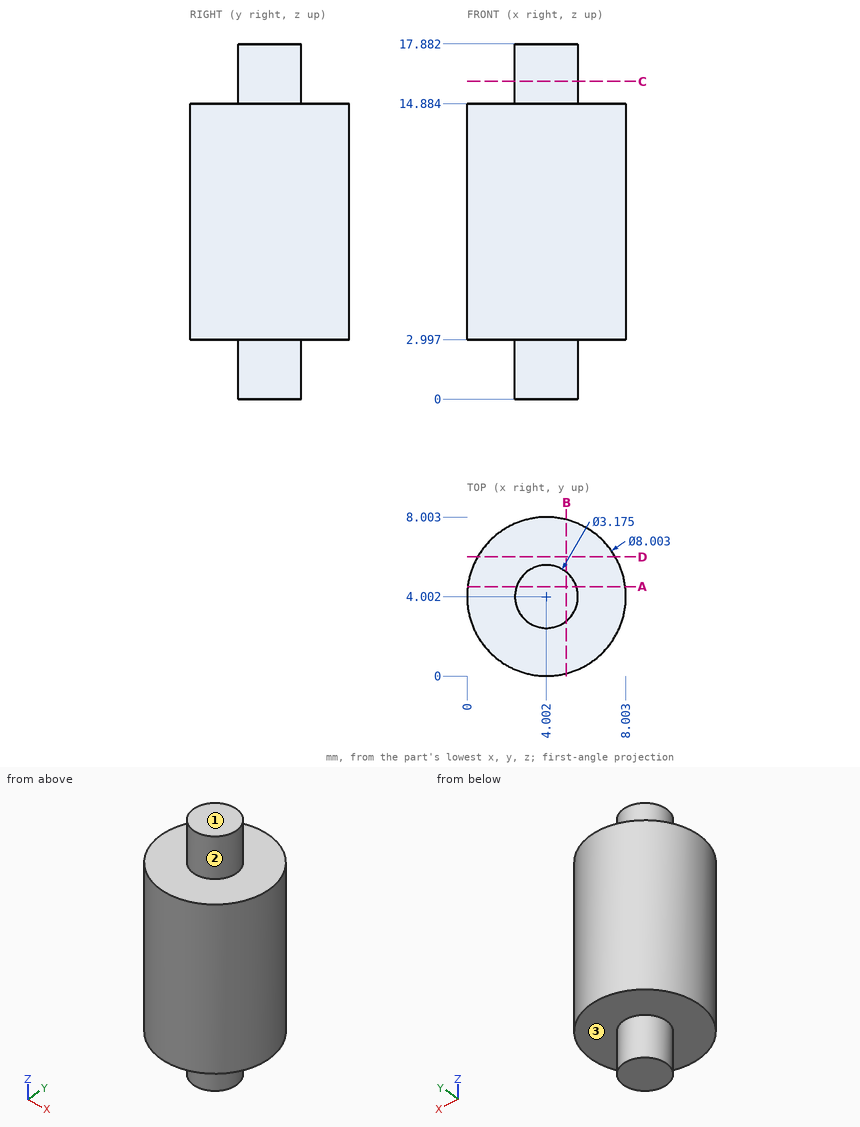
Verification items for this drawing (mm, ordinates from the low corner). A direction names the side the tool comes from. Round coordinates to 2 decimals unless told otherwise and drop trailing zeros. Loops run counter-clockwise (first coordinate to the right, second up) from the corner with the lowest first, then second, coordinate; pieces in that order, holes last. Notation, with made-up numbers: (50, 69.25) - (80, 69.25) arc R17 ccw to (80, 87.25) - close; hole circle Ø5 at (87.25, -32.5). An arc over 180 degrees is marked (long way). Write item = value, one per line.
Q1. Sectioned sample at A-A on y = 4.5. Record the boundary of the cut face in (x, z) (1 decimal).
Here are the results:
outline = (0, 3) - (2.5, 3) - (2.5, 0) - (5.5, 0) - (5.5, 3) - (8, 3) - (8, 14.9) - (5.5, 14.9) - (5.5, 17.9) - (2.5, 17.9) - (2.5, 14.9) - (0, 14.9) - close
Q2. Sectioned sample at D-D on y = 6. Record the boundary of the cut face in (x, z) (1 decimal).
Here are the results:
outline = (0.5, 3) - (7.5, 3) - (7.5, 14.9) - (0.5, 14.9) - close
Q3. Depth check by flat-ended pin: pin 1 (1 mm diameter, centred on y = 2, z = 10, fed in from -X); pin 2 (2 mm diameter, centred on x = 1, z = 6, fed in from +Y). Enter the tip coordinate at first touch or a pass-through.
Here are the results:
pin_1 = 0.29
pin_2 = 7.47
Q4. Sectioned sample at C-C on z = 16. Record the boundary of the cut face in (x, y) (1 decimal).
Here are the results:
outline = circle Ø3.2 at (4, 4)
Q5. Sectioned sample at B-B on x = 5. Record the boundary of the cut face in (y, z) (1 decimal), plus the area to 3 significant figures.
Here are the results:
outline = (0.1, 3) - (2.8, 3) - (2.8, 0) - (5.2, 0) - (5.2, 3) - (7.9, 3) - (7.9, 14.9) - (5.2, 14.9) - (5.2, 17.9) - (2.8, 17.9) - (2.8, 14.9) - (0.1, 14.9) - close
area = 107 mm^2
Q6. Tool access check on the marked faces 1, 2 and 3. Record the directions out of +Z, -Z, +X, -X, +Y, -Y that give a thin tool (end or side, any length) a straight path to the whole face; none if there is none.
Here are the results:
face_1 = +Z, +X, -X, +Y, -Y
face_2 = +Z
face_3 = -Z
Q7. Material ranges on L1, parallel to Z at x = 2, y = 5.75 (1 decimal); L2, parallel to X at y = 5.5, z = 12; L3, parallel to Y at x = 5.25, z = 7.5, recorded low to high.
Here are the results:
L1 = 3 to 14.9
L2 = 0.29 to 7.71
L3 = 0.2 to 7.8
